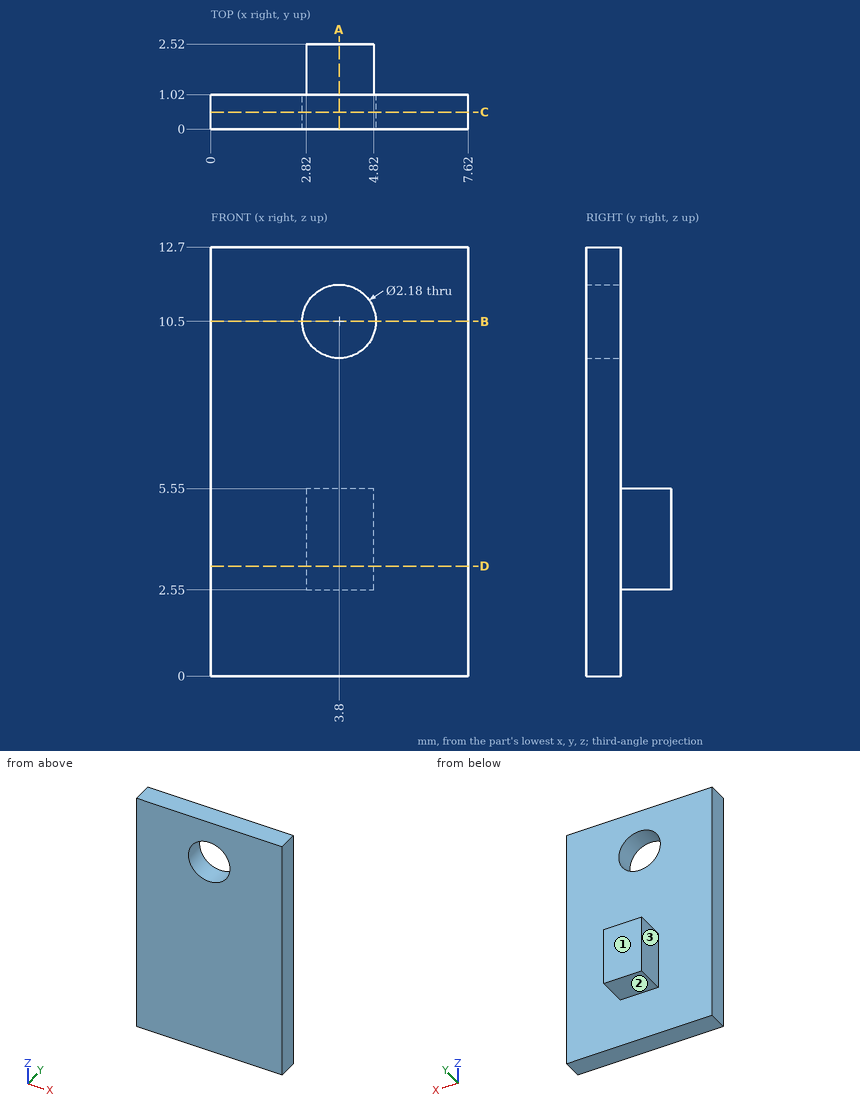
Input: dimensioned drawing with shaded views. Units: mm. Origin: part minimum x, y, z. A direction names the side the tool comes from. Coordinates: 2 decimals unless noted, no trailing zeros. Order: outer loops, then holes, each group sorted by start corner. A loop starts at its lowest first (then second) coordinate and runs counter-clockwise, first axis right, second up. Notation, with made-up numbers: (79.25, -22) - (135.25, -22) arc R9 ccw to (135.25, -12) - close; hole circle Ø4 at (69, 72). An arc over 180 degrees is marked (long way). Return JSON: item names as keys, results as strings. Group by question number.
1. Set-up query: the marked faces 1, 2 and 3. Return all of +Z, -Z, +X, -X, +Y, -Y with unobstructed straight access to the full face (end or side cutting, diameter ignored); none if empty.
2. Cut plane D-D (z = 3.25). Output: boundary loops of the cut face in (x, y).
3. Material intervals for line 1 along X through (y, z) = (0.75, 10.5); line 2 along Z through (x, y) = (3.8, 0.6); line 3 along Y through (x, z) = (4, 7.75), sorted ascending. Write a range as [from, to].
4. Pin query (flat end, axial travel): pin 1 (1.5 mm diameter, centred on x = 6, z = 5.5, fed in from +Y); pin 2 (1.2 mm diameter, centred on x = 3.5, y = 2, fed in from -Z); pin 3 (1.2 mm diameter, centred on y = 2, z = 4.5, fed in from -X). Return the tip coordinate at first contact, or that it passes through.
5. Cut plane A-A (x = 3.8). Output: boundary loops of the cut face in (y, z), plus the area to 3 significant figures.
6. Cut plane B-B (z = 10.5). Output: boundary loops of the cut face in (x, y).
7. Cut plane C-C (y = 0.5). Output: boundary loops of the cut face in (x, z), plus the area to 3 significant figures.
Resolved:
{
 "1": {"face 1": "+Z, -Z, +X, -X, +Y", "face 2": "-Z, +X, -X, +Y", "face 3": "+Z, -Z, -X, +Y"},
 "2": {"outline": "(0, 0) - (7.62, 0) - (7.62, 1.02) - (4.82, 1.02) - (4.82, 2.52) - (2.82, 2.52) - (2.82, 1.02) - (0, 1.02) - close"},
 "3": {"line 1": "x = [0, 2.71], [4.89, 7.62]", "line 2": "z = [0, 9.41], [11.59, 12.7]", "line 3": "y = [0, 1.02]"},
 "4": {"pin 1": "stops at y = 1.02", "pin 2": "stops at z = 2.55", "pin 3": "stops at x = 2.82"},
 "5": {"outline": "(0, 0) - (1.02, 0) - (1.02, 2.55) - (2.52, 2.55) - (2.52, 5.55) - (1.02, 5.55) - (1.02, 9.41) - (0, 9.41) - close; (0, 11.59) - (1.02, 11.59) - (1.02, 12.7) - (0, 12.7) - close", "area": "15.2 mm²"},
 "6": {"outline": "(0, 0) - (2.71, 0) - (2.71, 1.02) - (0, 1.02) - close; (4.89, 0) - (7.62, 0) - (7.62, 1.02) - (4.89, 1.02) - close"},
 "7": {"outline": "(0, 0) - (7.62, 0) - (7.62, 12.7) - (0, 12.7) - close; hole circle Ø2.18 at (3.8, 10.5)", "area": "93.0 mm²"}
}
